from build123d import *

# Parameters (mm, degrees)
F2_DEPTH = 26.75
F3_R     = 4


with BuildPart() as f2:
    # F1 (on Right) → F2 (new body, symmetric)
    with BuildSketch(Plane.YZ):
        Polygon((-19.3, 7), (-21.25, 0), (21.25, 0), (19.3, 7), align=None)
    extrude(amount=F2_DEPTH, both=True)

    # F3
    f3_edges = [f2.edges().sort_by_distance(p)[0] for p in [
        (-26.75, -20.275, 3.5),
        (26.75, -20.275, 3.5),
        (26.75, 20.275, 3.5),
        (-26.75, 20.275, 3.5),
    ]]
    fillet(f3_edges, radius=F3_R)


solid = f2.part
Check sheet for the modelled part. Datum: model origin and axes. Units: mm. Coordinates: 2 decimals unless noted, no trailing zeros. Loops run counter-clockwise (first coordinate to the right, second up) from the corner with the lowest first, then second, coordinate; pieces in that order, holes last. Notation, with made-up numbers: (-1, -18) -> (12, -18) arc R18 ccw to (12, 4) -> close; hole circle Ø6 at (-36.75, -30.75). An arc over 180 degrees is marked (long way). Write item = value, one per line. Start each with the question number.
1. Depth check by flat-ended pin: P1, Ø1, axis at x = 1, z = 1.5, coming from the -Y side; P2, Ø4, axis at x = 19, z = 1.5, coming from the +Y side. Enter the tip coordinate at first touch or a pass-through.
2. Section check A-A on x = -21. Record the cut outline in (y, z).
3. Material ranges on line 1 (Y direction, x = 7, z = 1.75); line 2 (Y direction, x = 18, z = 1.25); line 3 (X direction, y = -18.5, z = 6.25), recorded low to high.
Responses:
q1.P1 = -20.97
q1.P2 = 21.25
q2.outline = (-21.25, 0) -> (21.25, 0) -> (19.3, 7) -> (-19.3, 7) -> close
q3.line_1 = -20.76 to 20.76
q3.line_2 = -20.9 to 20.9
q3.line_3 = -25.36 to 25.36
